Work out the finished part from the listing and answer in its coordinate system (mm). A direction names the side the tool comes from. Coordinates: 2 decimals unless noted, no trailing zeros. Order: outer loops, then holes, each group sorted by start corner. A loop starts at its lowest first (then second) coordinate and runs counter-clockwise, first axis right, second up. Notation, with made-up numbers: (-2, 12) - (23, 12) arc R25 cw to (23, 43) - close; hole circle Ø10 at (89, -16). An arc over 180 degrees is marked (long way). Answer as a JSON object with one key per item and string values. Group by question number.
1) Section B-B (x = -20) is taken. Give the vertices of the cut face in (y, z), plus the area to 3 significant figures.
2) Section D-D (y = 3) is taken. Give the vertices of the cut face in (x, z).
3) A tool of negligible diameter and unlimited length cuts with its end or side. For faces 4 (the face through (2, 1.981, 13)), 5 (the face through (-35, -13.77, 12)), from which of +Z, -Z, +X, -X, +Y, -Y can it reach the whole face along a straight path? Write none if from no direction.
4) Each of these flat-tipped pins is pushed along its axis until it touches: P1, Ø8, axis at y = -4.5, z = 16, coming from the +X side; P2, Ø4, axis at x = -18.5, z = 21, coming from the -Y side. Where does it stop, or does it pass through?
5) Section C-C (z = 18.5) is taken. Give the vertices of the cut face in (x, y).
6) The mould has two halves that part along X. Classify faces 1 (the face through (38.563, 7, 12)), 2 (the face through (-12.196, 6.541, 12.173)), 3 (the face through (-2, 6, 25)): released by +X, released by -X, zero draft, split by the parting line, or undercut.
7) Section A-A (z = 14.75) is taken. Give the vertices of the cut face in (x, y), plus the area to 3 significant figures.
8) Find the intervals of material crossed by line 1 along Y through (x, z) = (-26, 14.5); line 2 along X through (y, z) = (-1.25, 10); line 3 along X through (y, z) = (4.25, 6.75), in increasing order.
from build123d import *

# Parameters (mm, degrees)
F0_W     = 75
F0_H     = 25
F1_DEPTH = 25
F2_W     = 71.5489391237
F2_H     = 15.7507188409
F3_DEPTH = 25
F4_R     = 5.3592968527
F5_DEPTH = 25


with BuildPart() as f1:
    # F0 (on Top) → F1 (new body)
    with BuildSketch(Plane.XY):
        with Locations((1.0630879551, -1.2695866427)):
            Rectangle(F0_W, F0_H)
    extrude(amount=F1_DEPTH)

    # F2 (on face) → F3 (cut)
    with BuildSketch(Plane.XY.offset(25)):
        with Locations((2.7886183932, -5.8942272223)):
            Rectangle(F2_W, F2_H)
    extrude(amount=-F3_DEPTH, mode=Mode.SUBTRACT)

    # F4 (on face) → F5 (cut)
    with BuildSketch(Plane.XZ.offset(-1.9811321981)):
        with Locations((-17.3081532121, 10.5629041791)):
            Circle(F4_R)
    extrude(amount=-F5_DEPTH, mode=Mode.SUBTRACT)


solid = f1.part
Report:
{
 "1": {"outline": "(1.98, 0) - (11.23, 0) - (11.23, 5.93) - (1.98, 5.93) - close; (1.98, 15.2) - (11.23, 15.2) - (11.23, 25) - (1.98, 25) - close", "area": "146 mm²"},
 "2": {"outline": "(-36.44, 0) - (38.56, 0) - (38.56, 25) - (-36.44, 25) - close; hole circle Ø10.72 at (-17.31, 10.56)"},
 "3": {"face 4": "+Z, -Z, +X, -Y", "face 5": "+Z, -Z, +X, -X, -Y"},
 "4": {"P1": "stops at x = -32.99", "P2": "stops at y = 1.98"},
 "5": {"outline": "(-36.44, -13.77) - (-32.99, -13.77) - (-32.99, 1.98) - (38.56, 1.98) - (38.56, 11.23) - (-36.44, 11.23) - close"},
 "6": {"face 1": "released by +X", "face 2": "undercut", "face 3": "zero draft"},
 "7": {"outline": "(-36.44, -13.77) - (-32.99, -13.77) - (-32.99, 1.98) - (-20.65, 1.98) - (-20.65, 11.23) - (-36.44, 11.23) - close; (-13.96, 1.98) - (38.56, 1.98) - (38.56, 11.23) - (-13.96, 11.23) - close", "area": "686 mm²"},
 "8": {"line 1": "y = 1.98 to 11.23", "line 2": "x = -36.44 to -32.99", "line 3": "x = -36.44 to -21.07, -13.54 to 38.56"}
}
